```python
from build123d import *

# Parameters (mm, degrees)
ESBO_O1_W                 = 100
ESBO_O1_H                 = 60
RESSALTO_EXTRUS_O1_DEPTH  = 9.525
FILETE1_R                 = 10
FURO_ROSCADO_DE_M61_D     = 5
FURO_ROSCADO_DE_M61_DEPTH = 15
FURO_ROSCADO_DE_M61_TIP   = 1.502151548
ESBO_O5_R                 = 3
CORTE_EXTRUS_O1_DEPTH     = 60.082363062
FURO_ROSCADO_DE_M82_D     = 6.8


with BuildPart() as part:
    # Esboço1 → Ressalto-extrusão1 (new body)
    with BuildSketch(Plane.XY):
        Rectangle(ESBO_O1_W, ESBO_O1_H)
    extrude(amount=RESSALTO_EXTRUS_O1_DEPTH)

    # Filete1
    filete1_edges = [part.edges().sort_by_distance(p)[0] for p in [
        (-50, 30, 4.7625),
        (50, 30, 4.7625),
    ]]
    fillet(filete1_edges, radius=FILETE1_R)

    # Furo roscado de M61
    with Locations(Plane(origin=(0, -30, 0), x_dir=(-1, 0, 0), z_dir=(0, -1, 0))):
        with Locations((20, -4.7625), (-20, -4.7625)):
            Hole(FURO_ROSCADO_DE_M61_D / 2, depth=FURO_ROSCADO_DE_M61_DEPTH)
            with Locations((0, 0, -(FURO_ROSCADO_DE_M61_DEPTH + FURO_ROSCADO_DE_M61_TIP / 2))):  # 118° drill point
                Cone(0, FURO_ROSCADO_DE_M61_D / 2, FURO_ROSCADO_DE_M61_TIP, mode=Mode.SUBTRACT)

    # Esboço5 → Corte-extrusão1 (cut, through all)
    with BuildSketch(Plane.XY.offset(9.525)):
        with Locations((30, -15)):
            Circle(ESBO_O5_R)
        with Locations((-30, -15)):
            Circle(ESBO_O5_R)
    extrude(amount=-CORTE_EXTRUS_O1_DEPTH, mode=Mode.SUBTRACT)

    # Furo roscado de M82 (through all)
    with Locations(Plane(origin=(30, -15, 0), x_dir=(-1, 0, 0), z_dir=(0, 0, -1))):
        with Locations((0, 0), (60, 0)):
            Hole(FURO_ROSCADO_DE_M82_D / 2)


solid = part.part
```
Check sheet for the modelled part. Datum: model origin and axes. Units: mm. A direction names the side the tool comes from. Coordinates: 2 decimals unless noted, no trailing zeros. Write each loop counter-clockwise with the first axis right and the second up, starting at its lowest first coordinate (ties: lowest second). Pieces come first, ordered by that corner, then holes. Notation, with made-up numbers: M 75,-34 L 90,-34 A14 ccw 90,-10 Z; hole C 1,41 d1. An arc over 180 degrees is marked long. Write item = value, one per line. Start each with the question number.
1. Go/stop test with flat-tipped pins: pin 1 (4.5 mm diameter, centred on x = 20, z = 4.76, fed in from -Y); pin 2 (3 mm diameter, centred on x = -20, z = 4.76, fed in from -Y). Record where each tip stops, or that it passes through.
2. Sectioned sample at B-B (x = 31.5). Record the cut outline in (y, z) (3 decimals).
3. Sectioned sample at A-A (x = -30). Record the cut outline in (y, z) (3 decimals).
4. Thickness scan on probe 1 along Z at (x, y) = (-20, -21) (1 decimal); probe 2 along X at (y, z) = (-14, 2); probe 3 along Y at (x, z) = (30, 6.5). Record the ranges inside material, lowest first.
5. Tool access check on faces 1 (the cylindrical face through (-22.5, -22.4, 4.7)), 2 (the cylindrical face through (33.14, -16.3, 4.83)). Record the directions out of +Z, -Z, +X, -X, +Y, -Y that give a thin tool (end or side, any length) a straight path to the whole face; none if there is none.
6. Mould release check, pull along Z, two halves, no side actions. Record for faces 3 (the flat face through (-1, 30, 5)), 4 (the flat face through (-1, 0, 9.525)), 5 (the conical face through (19.6, -13.76, 4.93)): pulls with the +Z half, pulls with the -Z half, needs draft (parallel to the pull), parting line crosses it, or undercut.
The answers:
q1.pin_1 = -14.85
q1.pin_2 = -14.4
q2.outline = M -30,0 L -18.051,0 L -18.051,9.525 L -30,9.525 Z; M -11.949,0 L 30,0 L 30,9.525 L -11.949,9.525 Z
q3.outline = M -30,0 L -18.4,0 L -18.4,9.525 L -30,9.525 Z; M -11.6,0 L 30,0 L 30,9.525 L -11.6,9.525 Z
q4.probe_1 = 0 to 2.3, 7.3 to 9.5
q4.probe_2 = -50 to -33.25, -26.75 to 26.75, 33.25 to 50
q4.probe_3 = -30 to -18.4, -11.6 to 30
q5.face_1 = -Y
q5.face_2 = +Z, -Z
q6.face_3 = needs draft
q6.face_4 = pulls with the +Z half
q6.face_5 = undercut
